from build123d import *

# Parameters (mm, degrees)
FILLET_1_R          = 0.2
CHAMFER_1_SIZE      = 0.2
SKETCH_3_W          = 0.5
SKETCH_3_H          = 0.25
CUT_EXTRUDE_1_DEPTH = 2


with BuildPart() as part:
    # 草图1 → 旋转1 (revolve)
    with BuildSketch(Plane.XY):
        Polygon((-6.5, 0), (-6.5, 3), (-3.5, 3), (-3.5, 1.5), (2.5, 1.5), (2.5, 1.25), (6.5, 1.25), (6.5, 0), align=None)
    revolve(axis=Axis((-6.5, 0, 0), (1, 0, 0)))

    # 圆角1
    fillet_1_edges = [part.edges().sort_by_distance(p)[0] for p in [
        (-3.5, -3, 0),
        (-6.5, -3, 0),
    ]]
    fillet(fillet_1_edges, radius=FILLET_1_R)

    # 倒角1
    chamfer_1_edges = [part.edges().sort_by_distance(p)[0] for p in [
        (6.5, -1.25, 0),
    ]]
    chamfer(chamfer_1_edges, length=CHAMFER_1_SIZE)

    # 草图3 → 切除-旋转1 (revolve, cut)
    with BuildSketch(Plane.XY):
        with Locations((2.75, 1.125)):
            Rectangle(SKETCH_3_W, SKETCH_3_H)
    revolve(axis=Axis((2.5, 0, 0), (1, 0, 0)), mode=Mode.SUBTRACT)

    # 草图4 → 切除-拉伸1 (cut)
    with BuildSketch(Plane.ZY.offset(6.5)):
        Polygon((1.732050808, 0), (0.866025404, 1.5), (-0.866025404, 1.5), (-1.732050808, 0), (-0.866025404, -1.5), (0.866025404, -1.5), align=None)
    extrude(amount=-CUT_EXTRUDE_1_DEPTH, mode=Mode.SUBTRACT)


solid = part.part
CAD build for the part. Positions are in the model's coordinates, mm. A direction names the side the tool comes from. Round coordinates to 2 decimals unless told otherwise and drop trailing zeros. Loops run counter-clockwise (first coordinate to the right, second up) from the corner with the lowest first, then second, coordinate; pieces in that order, holes last.
(1) Wall check: line 1 along X through (y, z) = (0.5, 2.25); line 2 along Z through (x, y) = (5, -0.75); line 3 along Z through (x, y) = (2.25, 0). Give the ranges that are in metal, low to high.
(2) Cut at B-B (z = 0). Give the cut face in (x, y), plus the area to 3 significant figures.
(3) Two-plate mould, pull along Z, no slides. Class faces 4 (the cylindrical face through (-5, -3, 0)), 5 (the flat face through (-3.5, 1.2, -1.2)), 6 (the flat face through (-5.514, 0.76, -1.293)): +Z half, -Z half, draft (parallel to the pull), parting line (faces both ways), or undercut.
(4) Cut at C-C (x = 2). Give the cut face in (y, z).
(5) Which spindle directions (+Z, -Z, +X, -X, +Y, -Y) get a long thin tool onto all of the face, cutting with end or side? Do faces 1 (the flat face through (-6, -1.5, 0)), 2 (the cylindrical face through (2.754, -0.217, -0.976)), 3 (the cylindrical face through (-0.46, -1.5, 0.07)). Say none if no direction does.
(6) Cut at A-A (x = -5). Give the cut face in (y, z), plus the area to 3 significant figures.
(7) Drop flat-ended pins along their axis: pin 1 (1.5 mm diameter, centred on y = 0.5, z = 0, fed in from -X); pin 2 (3 mm diameter, centred on y = 0.5, z = 0.5, fed in from -X); pin 3 (1.5 mm diameter, centred on x = -3, z = 0.5, fed in from -Y); pin 4 (3 mm diameter, centred on x = 1, z = 1, fed in from -Y). Give the stop position or say it passes through.
Findings below:
1. line 1: x = -6.5 to -3.5
1. line 2: z = -1 to 1
1. line 3: z = -1.5 to 1.5
2. outline: (-6.5, -2.8) arc R0.2 ccw to (-6.3, -3) - (-3.7, -3) arc R0.2 ccw to (-3.5, -2.8) - (-3.5, -1.5) - (2.5, -1.5) - (2.5, -1) - (3, -1) - (3, -1.25) - (6.3, -1.25) - (6.5, -1.05) - (6.5, 1.05) - (6.3, 1.25) - (3, 1.25) - (3, 1) - (2.5, 1) - (2.5, 1.5) - (-3.5, 1.5) - (-3.5, 2.8) arc R0.2 ccw to (-3.7, 3) - (-6.3, 3) arc R0.2 ccw to (-6.5, 2.8) - (-6.5, 1.5) - (-4.5, 1.5) - (-4.5, -1.5) - (-6.5, -1.5) - close
2. area: 39.7 mm2
3. face 4: parting line
3. face 5: draft
3. face 6: undercut
4. outline: circle Ø3 at (0, 0)
5. face 1: -X
5. face 2: none
5. face 3: +X
6. outline: circle Ø6 at (0, 0); hole (-1.5, -0.87) - (0, -1.73) - (1.5, -0.87) - (1.5, 0.87) - (0, 1.73) - (-1.5, 0.87) - close
6. area: 20.5 mm2
7. pin 1: stops at x = -4.5
7. pin 2: stops at x = -6.5
7. pin 3: stops at y = -2.99
7. pin 4: stops at y = -1.5
